Solid Edge part; units mm, degrees
sketch "Sketch1" plane through (5.8669, 0, 0) normal (1, 0, 0) x (0, 1, 0)
  arc A0 (-11.9528, 0) -> (-17.9528, 0) centre (-14.9528, 0) cw
  line L0 (-17.9528, 0) -> (-17.9528, 2.9)
  line L1 (-17.9528, 2.9) -> (-26.9528, 2.9)
  line L2 (-26.9528, 2.9) -> (-26.9528, -5.1)
  line L3 (-26.9528, -5.1) -> (27.0472, -5.1)
  line L4 (27.0472, -5.1) -> (27.0472, 2.9)
  line L5 (27.0472, 2.9) -> (18.0472, 2.9)
  line L6 (18.0472, 0) -> (18.0472, 2.9)
  arc A1 (18.0472, 0) -> (12.0472, 0) centre (15.0472, 0) cw
  line L7 (12.0472, 0) -> (12.0472, 2.9)
  line L8 (12.0472, 2.9) -> (-11.9528, 2.9)
  line L9 (-11.9528, 0) -> (-11.9528, 2.9)
extrude "Protrusion1" add sketch "Sketch1" along normal up to vertex (10 mm away)
sketch "Sketch2" plane through (10.8669, 0.0472, -5.1) normal (0, 0, -1) x (0, 1, 0)
  circle A0 centre (-23.254, 0.6696) radius 1.7
  circle A1 centre (0, 0.6696) radius 1.2295
  circle A2 centre (23.254, 0.6696) radius 1.7
extrude "Cutout1" cut sketch "Sketch2" against normal up to next
properties material "ABS Plastic, high impact"
The model under review builds one solid part; all positions refer to its coordinate system, in mm. A direction names the side the tool comes from. Give positions to 0.01 mm unless a question says otherwise; leave off trailing zeros. Write each loop counter-clockwise with the first axis right and the second up, starting at its lowest first coordinate (ties: lowest second). Pieces come first, ordered by that corner, then holes. Notation, with made-up numbers: (-22.5, 47) - (9.5, 47) arc R16 ccw to (9.5, 78) - close; hole circle Ø3 at (-37, 6.25). An arc over 180 degrees is marked (long way). Answer in a Markdown table with one row per item. Add a question column.
1. We need section A-A on z = 0.75. Write out the cut boundary in (x, y).
2. We need section D-D on y = 16. Write out the cut boundary in (x, z).
3. We need section B-B on x = 12. Write out the cut boundary in (y, z).
4. Tool access review of faces 1 (the flat face through (11, -21, 2.9)), 2 (the flat face through (11, 12.047, 1)): name each direction out of +Z, -Z, +X, -X, +Y, -Y from which nothing blocks a thin tool from reaching the whole face with its end or side.
5. We need section C-C on z = -2. Write out the cut boundary in (x, y).
6. Draft analysis for pull direction Y (two halves, no side actions). For faces 3 (the flat face through (10, 0, 2.9)), 4 (the flat face through (11, 27.047, -1)), 5 (the flat face through (11, 18.047, 1)), state which applies: +Y half, -Y half, draft (parallel to the pull), parting line (faces both ways), or undercut.
7. Wall thickness on line 1 along Y through (x, z) = (14, 1.5); line 2 along Y through (x, z) = (13.5, -0.25); line 3 along Y through (x, z) = (10.75, -3.25): over which ranges is each line inside the solid? List them lowest first. Write a range as [from, to].
Ans:
| question | item | result |
|---|---|---|
| 1 | outline | (5.87, -26.95) - (15.87, -26.95) - (15.87, -17.95) - (5.87, -17.95) - close; (5.87, -11.95) - (15.87, -11.95) - (15.87, 12.05) - (5.87, 12.05) - close; (5.87, 18.05) - (15.87, 18.05) - (15.87, 27.05) - (5.87, 27.05) - close; hole circle Ø3.4 at (11.54, -23.21); hole circle Ø3.4 at (11.54, 23.3); hole circle Ø2.46 at (11.54, 0.05) |
| 2 | outline | (5.87, -5.1) - (15.87, -5.1) - (15.87, -2.84) - (5.87, -2.84) - close |
| 3 | outline | (-26.95, -5.1) - (-24.84, -5.1) - (-24.84, 2.9) - (-26.95, 2.9) - close; (-21.57, -5.1) - (-1.09, -5.1) - (-1.09, 2.9) - (-11.95, 2.9) - (-11.95, 0) arc R3 cw to (-17.95, 0) - (-17.95, 2.9) - (-21.57, 2.9) - close; (1.19, -5.1) - (21.67, -5.1) - (21.67, 2.9) - (18.05, 2.9) - (18.05, 0) arc R3 cw to (12.05, 0) - (12.05, 2.9) - (1.19, 2.9) - close; (24.94, -5.1) - (27.05, -5.1) - (27.05, 2.9) - (24.94, 2.9) - close |
| 4 | face 1 | +Z, +X, -X, +Y, -Y |
| 4 | face 2 | +Z, +X, -X |
| 5 | outline | (5.87, -26.95) - (15.87, -26.95) - (15.87, -17.19) - (5.87, -17.19) - close; (5.87, -12.72) - (15.87, -12.72) - (15.87, 12.81) - (5.87, 12.81) - close; (5.87, 17.28) - (15.87, 17.28) - (15.87, 27.05) - (5.87, 27.05) - close; hole circle Ø3.4 at (11.54, -23.21); hole circle Ø3.4 at (11.54, 23.3); hole circle Ø2.46 at (11.54, 0.05) |
| 6 | face 3 | draft |
| 6 | face 4 | +Y half |
| 6 | face 5 | undercut |
| 7 | line 1 | y = [-26.95, -17.95], [-11.95, 12.05], [18.05, 27.05] |
| 7 | line 2 | y = [-26.95, -17.94], [-11.96, 12.06], [18.04, 27.05] |
| 7 | line 3 | y = [-26.95, -24.71], [-21.7, -0.9], [0.99, 21.79], [24.81, 27.05] |
